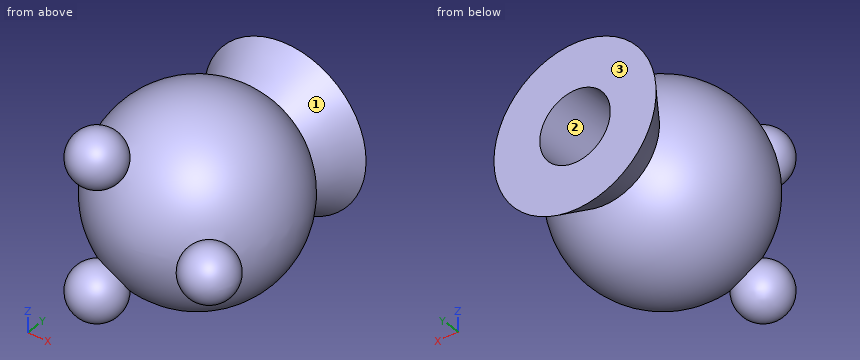
```python
from build123d import *

# Parameters (mm, degrees)
CIRPATTERN1_COUNT = 3


with BuildPart() as part:
    # Sketch1 → Revolve1 (revolve)
    with BuildSketch(Plane.XY):
        with BuildLine():
            Line((0, 0), (0, 40))
            Line((0, 40), (10, 40))
            Line((10, 40), (10, 60))
            Line((10, 60), (23, 60))
            Line((23, 60), (15.652475842, 49))
            ThreePointArc((15.652475842, 49), (25.719642299, 18.784161637), (0, 0))
        make_face()
    revolve(axis=Axis((0, 0, 0), (0, 1, 0)))

    # Sketch2 → Revolve2 (revolve)
    with BuildSketch(Plane.XY):
        with BuildLine():
            Line((15.909902577, 8.590097423), (26.516504294, -2.016504294))
            ThreePointArc((26.516504294, -2.016504294), (26.516504294, 8.590097423), (15.909902577, 8.590097423))
        make_face()
    revolve2 = revolve(axis=Axis((15.909902577, 8.590097423, 0), (0.707106781186544, -0.7071067811865511, 0)))

    # CirPattern1: Revolve2 ×3 about axis
    cirpattern1_axis = Axis((0, 0, 0), (0, 1, 0))
    for i in range(1, CIRPATTERN1_COUNT):
        add(revolve2.rotate(cirpattern1_axis, i * 360 / CIRPATTERN1_COUNT))


solid = part.part
```
Here's how the part is built. I have some questions about the finished solid (model axes, mm). Face numbers are marked on the shaded views. Coordinates: 2 decimals unless noted, no trailing zeros. Loops run counter-clockwise (first coordinate to the right, second up) from the corner with the lowest first, then second, coordinate; pieces in that order, holes last. Notation, with made-up numbers: (-3, 1.25) -> (19, 1.25) arc R18 cw to (19, 15.25) -> close; hole circle Ø2 at (15, 35.5). An arc over 180 degrees is marked (long way). Return JSON: item names as keys, results as strings.
1) If we section it at D-D, the plane x = -17: Count the separate pieces of the cut face and the enclosed holes in it, then the cut area to 3 significant figures.
Results below:
{"separate pieces": "4", "enclosed holes": "0", "area": "1,660 mm²"}
2) Will these pins go through, and if not, where does the flat tip stop? pin 1 (4 mm diameter, centred on y = 39.5, z = 21.5, fed in from +X); pin 2 (6 mm diameter, centred on x = 0, z = 0.5, fed in from +Y); pin 3 (23 mm diameter, centred on x = 0, z = 0, fed in from -Y).
Results below:
{"pin 1": "x = 14.35", "pin 2": "y = 40", "pin 3": "y = 0"}
3) If we section it at C-C, the plane x = 0: Write out the boundary of the cut face in (y, z).
Results below:
{"outline": "(40, -10) -> (40, 10) -> (60, 10) -> (60, 23) -> (49, 15.65) arc R27 ccw (long way) to (49, -15.65) -> (60, -23) -> (60, -10) -> close"}
4) If we section it at B-B, the plane y = 5: Write out the boundary of the cut face in (x, z), then the cut area to 3 significant figures.
Results below:
{"outline": "(-11.05, -11.08) arc R7.3 ccw (long way) to (-4.07, -15.11) arc R15.65 ccw to (15.12, -4.03) arc R7.3 ccw (long way) to (15.12, 4.03) arc R15.65 ccw to (-4.07, 15.11) arc R7.3 ccw (long way) to (-11.05, 11.08) arc R15.65 ccw to start", "area": "1,240 mm²"}
5) Thinking about a two-plate mould opening in Y: for the marked faces 1, 2 and 3, which applies, +Y half, -Y half, draft (parallel to the pull), parting line (faces both ways), or undercut?
Results below:
{"face 1": "undercut", "face 2": "draft", "face 3": "+Y half"}
6) I need wall thicknesses on line 1 (X direction, y = 53.75, z = 0); line 2 (X direction, y = 51, z = 0); line 3 (Z direction, x = -14.5, y = 0). Which ranges of each line are inside material? Lowest first, please. Write a range as from..to.
Results below:
{"line 1": "-18.83..-10, 10..18.83", "line 2": "-16.99..-10, 10..16.99", "line 3": "-23.87..-12.87, 12.87..23.87"}
7) If we section it at A-A, the plane z = 0: Write out the boundary of the cut face in (x, y), then the cut area to 3 significant figures.
Results below:
{"outline": "(-23, 60) -> (-15.65, 49) arc R27 ccw to (13.73, 3.75) arc R7.5 ccw (long way) to (21.58, 10.78) arc R27 ccw to (15.65, 49) -> (23, 60) -> (10, 60) -> (10, 40) -> (-10, 40) -> (-10, 60) -> close", "area": "2,370 mm²"}
